The model under review builds one solid part; all positions refer to its coordinate system, in mm. Coordinates: 2 decimals unless noted, no trailing zeros. Write each loop counter-clockwise with the first axis right and the second up, starting at its lowest first coordinate (ties: lowest second). Pieces come first, ordered by that corner, then holes. Notation, with made-up numbers: (56, 54.5) -> (114, 54.5) arc R29 ccw to (114, 87.5) -> close; hole circle Ø11 at (52, 22). An arc over 180 degrees is marked (long way). Put each result on its own line as item: value. Start each with the question number.
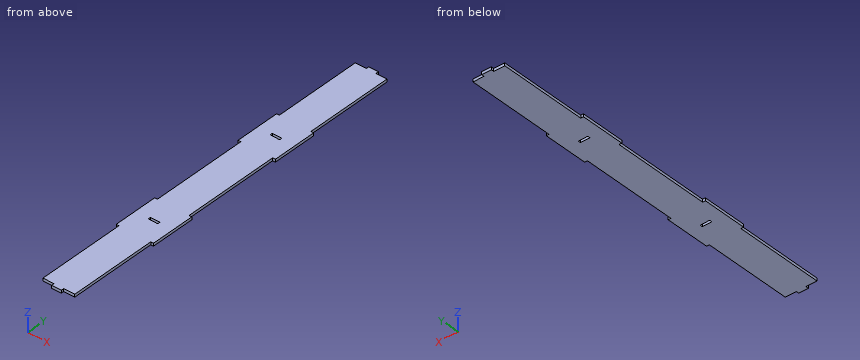
from build123d import *

# Parameters (mm, degrees)
SKETCH2_W           = 15
SKETCH2_H           = 4
BOSS_EXTRUDE1_DEPTH = 4.3


with BuildPart() as part:
    # Sketch2 → Boss-Extrude1 (new body)
    with BuildSketch(Plane.XY):
        Polygon((-25, -286), (-7.65, -286), (-7.65, -290.3), (7.65, -290.3), (7.65, -286), (25, -286), (25, -146.7666), (29.3, -146.7666), (29.3, -76.5666), (25, -76.5666), (25, 76.5667), (29.3, 76.5667), (29.3, 146.7667), (25, 146.7667), (25, 286), (7.65, 286), (7.65, 290.3), (-7.65, 290.3), (-7.65, 286), (-25, 286), (-25, 146.7667), (-29.3, 146.7667), (-29.3, 76.5667), (-25, 76.5667), (-25, -76.5666), (-29.3, -76.5666), (-29.3, -146.7666), (-25, -146.7666), align=None)
        with Locations((0, 111.6666)):
            Rectangle(SKETCH2_W, SKETCH2_H, mode=Mode.SUBTRACT)
        with Locations((0, -111.6666)):
            Rectangle(SKETCH2_W, SKETCH2_H, mode=Mode.SUBTRACT)
    extrude(amount=BOSS_EXTRUDE1_DEPTH)


solid = part.part
1. Insertion check: P1, Ø1.3, axis at x = 18, z = 2, coming from the -Y side; P2, Ø1.3, axis at y = -287, z = 1, coming from the -X side; P3, Ø2, axis at x = -28, z = 1, coming from the -Y side. Each pin has a flat end and moves straight along its axis. Give the tip position at first contact, or say it passes through.
2. Wall thickness on line 1 (Y direction, x = -2.5, z = 1.15); line 2 (X direction, y = -180.5, z = 1.7); line 3 (Y direction, x = -8, z = 1.6): over which ranges is each line inside the solid? List them lowest first. Write a range as from..to.
3. Consider section B-B on y = -24.5. State the section outline as (x, z) points, then the cut area to 3 significant figures.
4. Consider section A-A on z = 3. State how many separate pieces and enclosed holes the cut face has, then the cut area to 3 significant figures.
Output values:
1. P1: stops at y = -286
1. P2: stops at x = -7.65
1. P3: stops at y = -146.77
2. line 1: y = -290.3..-113.67, -109.67..109.67, 113.67..290.3
2. line 2: x = -25..25
2. line 3: y = -286..286
3. outline: (-25, 0) -> (25, 0) -> (25, 4.3) -> (-25, 4.3) -> close
3. area: 215 mm^2
4. separate pieces: 1
4. enclosed holes: 2
4. area: 29,800 mm^2
